The model under review builds one solid part; all positions refer to its coordinate system, in mm. Round coordinates to 2 decimals unless told otherwise and drop trailing zeros. Write each loop counter-clockwise with the first axis right and the second up, starting at its lowest first coordinate (ties: lowest second). Pieces come first, ordered by that corner, then holes.
Item 1: Add section B-B (x = 8.25). Give the boundary of the cut face in (y, z).
Item 2: Clearance check with flat-ended pins moving along their axes: pin 1 Ø1.5 at (x, z) = (10, -36.5) entering from -Y; pin 2 Ø1 at (x, y) = (10.5, 2.5) entering from -Z. State where each tip first meets the part, or that it passes through.
Item 3: To check wall thickness, follow L1, parallel to Z at x = 10.75, y = 0.85; L2, parallel to Z at x = 4.5, y = 4.2; L3, parallel to X at y = 3.8, z = -6. State the ranges of each line that lie inside material, in increasing order.
Item 4: Add section A-A (y = 2.55). State how many separate pieces and enclosed holes the cut face has, plus the area to 3 significant figures.
Item 5: Add section D-D (z = -9). Give the boundary of the cut face in (x, y), plus the area to 3 significant figures.
Item 6: Add section C-C (z = -37). Give the boundary of the cut face in (x, y), plus the area to 3 significant figures.
Item 7: Draft analysis for pull direction Z (two halves, no side actions). For faces 1 (the face through (15, 3, -21)), 2 (the face through (12.745, 3.042, -40.861)), 3 (the face through (5.1, 3, -10.2)), state which applies: +Z half, -Z half, draft (parallel to the pull), parting line (faces both ways), or undercut.
```python
from build123d import *

# Parameters (mm, degrees)
SKETCH1_W           = 15
SKETCH1_H           = 43
BOSS_EXTRUDE1_DEPTH = 6
SKETCH4_R           = 4
CUT_EXTRUDE2_DEPTH  = 46.934736311
FILLET1_R           = 7.5


with BuildPart() as part:
    # Sketch1 → Boss-Extrude1 (new body)
    with BuildSketch(Plane(origin=(0, 0, 0), x_dir=(1, 0, 0), z_dir=(0, 1, 0))):
        with Locations((7.5, 21.5)):
            Rectangle(SKETCH1_W, SKETCH1_H)
    extrude(amount=BOSS_EXTRUDE1_DEPTH)

    # Sketch4 → Cut-Extrude2 (cut, through all)
    with BuildSketch(Plane(origin=(0, 6, 0), x_dir=(1, 0, 0), z_dir=(0, 1, 0))):
        with Locations(Location((7.5, 37, 0), (0, 0, 270))):
            Circle(SKETCH4_R)
        with Locations(Location((7.5, 7, 0), (0, 0, 270))):
            Circle(SKETCH4_R)
    extrude(amount=-CUT_EXTRUDE2_DEPTH, mode=Mode.SUBTRACT)

    # Fillet1
    fillet1_edges = [part.edges().sort_by_distance(p)[0] for p in [
        (0, 3, 0),
        (15, 3, 0),
        (15, 3, -43),
        (0, 3, -43),
    ]]
    fillet(fillet1_edges, radius=FILLET1_R - 0.0001)  # a hair under: the kernel refuses the full size


solid = part.part
```
Numbers:
1. outline: (0, -42.96) - (6, -42.96) - (6, -40.93) - (0, -40.93) - close; (0, -33.07) - (6, -33.07) - (6, -10.93) - (0, -10.93) - close; (0, -3.07) - (6, -3.07) - (6, -0.04) - (0, -0.04) - close
2. pin 1: passes through
2. pin 2: stops at z = -42.57
3. L1: z = -42.26 to -39.33, -34.67 to -9.33, -4.67 to -0.74
3. L2: z = -42.37 to -39.65, -34.35 to -9.65, -4.35 to -0.63
3. L3: x = 0.15 to 3.63, 11.37 to 14.85
4. separate pieces: 1
4. enclosed holes: 2
4. area: 496 mm2
5. outline: (0, 0) - (4.04, 0) - (4.04, 6) - (0, 6) - close; (10.96, 0) - (15, 0) - (15, 6) - (10.96, 6) - close
5. area: 48.4 mm2
6. outline: (0.15, 0) - (3.5, 0) - (3.5, 6) - (0.15, 6) - close; (11.5, 0) - (14.85, 0) - (14.85, 6) - (11.5, 6) - close
6. area: 40.2 mm2
7. face 1: draft
7. face 2: -Z half
7. face 3: undercut
